```python
from build123d import *

# Parameters (mm, degrees)
BOSS_EXTRUDE2_DEPTH     = 58
SKETCH6_R               = 2.5
SKETCH6_R_2             = 20
CUT_EXTRUDE3_DEPTH      = 58
SKETCH7_R               = 1.5
CUT_EXTRUDE4_DEPTH      = 58
CUT_EXTRUDE4_DEPTH_BACK = 58


with BuildPart() as part:
    # Sketch5 → Boss-Extrude2 (new body)
    with BuildSketch(Plane(origin=(0, 0, 0), x_dir=(0, 0, -1), z_dir=(1, 0, 0))):
        with BuildLine():
            Line((108, 0), (108, -5))
            Line((108, -5), (31.304951685, -5))
            ThreePointArc((31.304951685, -5), (34.8658518, -7.764428241), (38.183766184, -10.816233816))
            Line((38.183766184, -10.816233816), (34.648232278, -14.351767722))
            ThreePointArc((34.648232278, -14.351767722), (18.751488186, -3.729902907), (0, 0))
            ThreePointArc((0, 0), (-18.751488186, -3.729902907), (-34.648232278, -14.351767722))
            Line((-34.648232278, -14.351767722), (-38.183766184, -10.816233816))
            ThreePointArc((-38.183766184, -10.816233816), (-20.664905348, 0.889494756), (0, 5))
            ThreePointArc((0, 5), (11.618950039, 3.735187494), (22.693611436, 0))
            Line((22.693611436, 0), (108, 0))
        make_face()
    extrude(amount=BOSS_EXTRUDE2_DEPTH)

    # Sketch6 → Cut-Extrude3 (cut)
    with BuildSketch(Plane(origin=(0, 0, 0), x_dir=(1, 0, 0), z_dir=(0, 1, 0))):
        with Locations((5.5, 102.5)):
            Circle(SKETCH6_R)
        with Locations((52.5, 102.5)):
            Circle(SKETCH6_R)
        with Locations((52.5, 55.5)):
            Circle(SKETCH6_R)
        with Locations((5.5, 55.5)):
            Circle(SKETCH6_R)
        with Locations((29, 79)):
            Circle(SKETCH6_R_2)
    extrude(amount=-CUT_EXTRUDE3_DEPTH, mode=Mode.SUBTRACT)

    # Sketch7 → Cut-Extrude4 (cut, two sides)
    with BuildSketch(Plane(origin=(0, 0, 0), x_dir=(1, 0, 0), z_dir=(0, 1, 0))) as cut_extrude4_sk:
        with Locations((15, 0)):
            Circle(SKETCH7_R)
        with Locations((43, 0)):
            Circle(SKETCH7_R)
    extrude(amount=CUT_EXTRUDE4_DEPTH, mode=Mode.SUBTRACT)
    extrude(cut_extrude4_sk.sketch, amount=-CUT_EXTRUDE4_DEPTH_BACK, mode=Mode.SUBTRACT)


solid = part.part
```
Part model, mm, in its own coordinate system. A direction names the side the tool comes from. Give positions to 0.01 mm unless a question says otherwise; leave off trailing zeros. Order: outer loops, then holes, each group sorted by start corner. A loop starts at its lowest first (then second) coordinate and runs counter-clockwise, first axis right, second up. Notation, with made-up numbers: (58, 28.5) - (99, 28.5) arc R17 ccw to (99, 42.5) - close; hole circle Ø11 at (-16, 83.5). An arc over 180 degrees is marked (long way). Use one line per item in the form item = value.
Item 1: Slice it at B-B on z = -102.5. Give the cut face in (x, y), and give its area (3 significant figures).
Solution:
outline = (0, -5) - (3, -5) - (3, 0) - (0, 0) - close; (8, -5) - (50, -5) - (50, 0) - (8, 0) - close; (55, -5) - (58, -5) - (58, 0) - (55, 0) - close
area = 240 mm2
Item 2: Which spindle directions (+Z, -Z, +X, -X, +Y, -Y) get a long thin tool onto all of the face, cutting with end or side? Do faces 1 (the face through (29, 0, -55)), 2 (the face through (0, -3, -35)), 3 (the face through (29, -5, -53)). Say none if no direction does.
Solution:
face_1 = -Z, +X, -X, +Y
face_2 = +Z, -Z, -X, +Y, -Y
face_3 = -Z, +X, -X
Item 3: Slice it at A-A on x = 5.5. Give the cut face in (y, z).
Solution:
outline = (-14.35, -34.65) - (-10.82, -38.18) arc R54 ccw to (-5, -31.3) - (-5, -53) - (0, -53) - (0, -22.69) arc R54 ccw to (-10.82, 38.18) - (-14.35, 34.65) arc R49 cw to start; (-5, -108) - (0, -108) - (0, -105) - (-5, -105) - close; (-5, -100) - (0, -100) - (0, -58) - (-5, -58) - close
Item 4: Two-plate mould, pull along Z, no slides. Class faces 4 (the face through (13.5, 2.45, -0.07)), 5 (the face through (58, -3, -35)), 6 (the face through (29, -13, 36)), 7 (the face through (54.81, -2.46, -54.54)): released by +Z, released by -Z, zero draft, split by the parting line, or undercut.
Solution:
face_4 = undercut
face_5 = zero draft
face_6 = released by +Z
face_7 = undercut
Item 5: Slice it at C-C on x = 29. Give the cut face in (y, z), and give its area (3 significant figures).
Solution:
outline = (-14.35, -34.65) - (-10.82, -38.18) arc R54 ccw to (-5, -31.3) - (-5, -59) - (0, -59) - (0, -22.69) arc R54 ccw to (-10.82, 38.18) - (-14.35, 34.65) arc R49 cw to start; (-5, -108) - (0, -108) - (0, -99) - (-5, -99) - close
area = 608 mm2
Item 6: Pin check, flat tips, straight feed: pin 1 Ø1 at (x, y) = (28, -10) entering from -Z; pin 2 Ø8 at (x, z) = (52.5, -55.5) entering from +Y; pin 3 Ø4 at (x, z) = (43, 0) entering from -Y; pin 4 Ø24 at (x, z) = (29, -79) entering from +Y (3 decimals). Stop position of each tip, or through.
Solution:
pin_1 = -37.86
pin_2 = 0
pin_3 = -0.04
pin_4 = through
Item 7: Slice it at D-D on y = 2. Give the cut face in (x, z).
Solution:
outline = (0, -17.75) - (58, -17.75) - (58, 17.75) - (0, 17.75) - close; hole circle Ø3 at (15, 0); hole circle Ø3 at (43, 0)
Item 8: Probe probe 1 along X at (y, z) = (2.8, 0); probe 2 along X at (y, z) = (-1.3, -55.5); probe 3 along Z at (x, y) = (43, -4). List the from-to ranges inside material, lowest first. Write a range as from..to.
Solution:
probe_1 = 0..13.5, 16.5..41.5, 44.5..58
probe_2 = 0..3, 8..50, 55..58
probe_3 = -108..-93.28, -64.72..-19.39, 19.39..29.85
